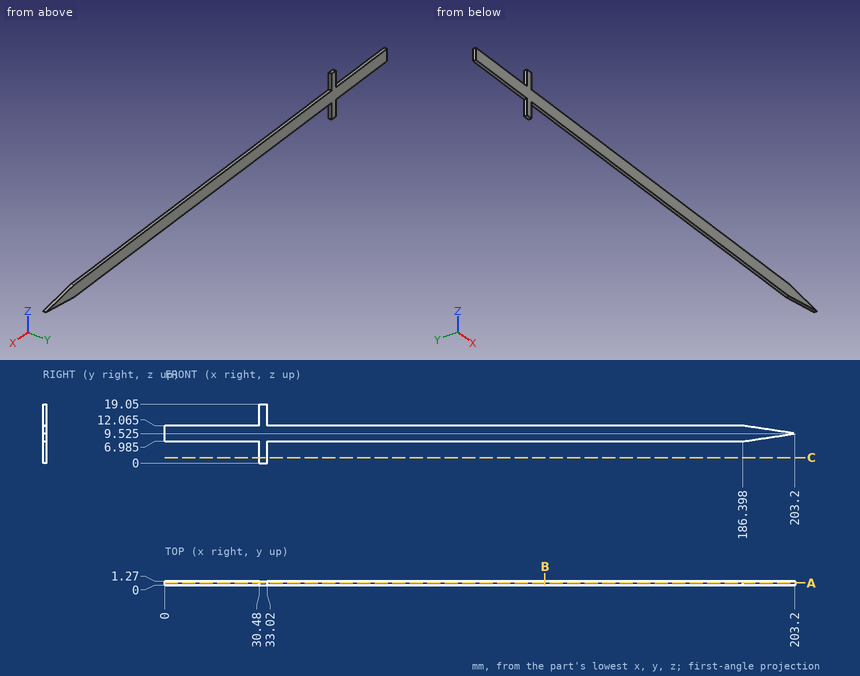
Design review of the part shown in the three views and the two pictorial views. Dimensions are in mm from the part's minimum x, y and z. Round coordinates to 2 decimals unless told otherwise and drop trailing zeros. Write each loop counter-clockwise with the first axis right and the second up, starting at its lowest first coordinate (ties: lowest second). Pieces come first, ordered by that corner, then holes. Notation, with made-up numbers: (58, 67.25) -> (110, 67.25) arc R21 ccw to (110, 87.25) -> close; hole circle Ø11 at (-32.5, 3.25). An arc over 180 degrees is marked (long way). Answer as a JSON object with one key per item and string values.
1. Clearance check with a flat-ended pin moving along its axis: pin 1 (0.6 mm diameter, centred on x = 83, y = 1, fed in from -Z) (3 decimals). State where the tip first meets the part, or that it passes through.
Results found:
{"pin 1": "stops at z = 6.985"}
2. We need section C-C on z = 1.75. State the section outline as (x, y) points.
Results found:
{"outline": "(30.48, 0) -> (33.02, 0) -> (33.02, 1.27) -> (30.48, 1.27) -> close"}
3. We need section B-B on x = 122.5. State the section outline as (y, z) points (3 decimals).
Results found:
{"outline": "(0, 6.985) -> (1.27, 6.985) -> (1.27, 12.065) -> (0, 12.065) -> close"}
4. To check wall thickness, follow line 1 along Z through (x, y) = (48, 1) (3 decimals); line 2 along X through (y, z) = (0.7, 4.25). State the ranges of each line that lie inside material, in increasing order.
Results found:
{"line 1": "z = 6.985 to 12.065", "line 2": "x = 30.48 to 33.02"}
5. We need section A-A on y = 0.65. State the section outline as (x, z) points (3 decimals).
Results found:
{"outline": "(0, 6.985) -> (30.48, 6.985) -> (30.48, 0) -> (33.02, 0) -> (33.02, 6.985) -> (186.398, 6.985) -> (203.2, 9.525) -> (186.398, 12.065) -> (33.02, 12.065) -> (33.02, 19.05) -> (30.48, 19.05) -> (30.48, 12.065) -> (0, 12.065) -> close"}
